```python
from build123d import *

# Parameters (mm, degrees)
EXTRUDE1_DEPTH     = 23.8125
SKETCH8_R          = 3.5687
CUT_EXTRUDE7_DEPTH = 73.566916507
SKETCH9_R          = 3.5687
CUT_EXTRUDE8_DEPTH = 73.566916507


with BuildPart() as part:
    # Sketch1 → Extrude1 (new, symmetric)
    with BuildSketch(Plane.XY):
        with BuildLine():
            Line((0, 0), (0, 50.8))
            ThreePointArc((0, 50.8), (-3.376576302, 49.401376302), (-4.7752, 46.0248))
            Line((-4.7752, 46.0248), (-4.7752, 8.3566))
            ThreePointArc((-4.7752, 8.3566), (-5.824167774, 5.824167774), (-8.3566, 4.7752))
            Line((-8.3566, 4.7752), (-46.0248, 4.7752))
            ThreePointArc((-46.0248, 4.7752), (-49.401376302, 3.376576302), (-50.8, 0))
            Line((-50.8, 0), (0, 0))
        make_face()
    extrude(amount=EXTRUDE1_DEPTH, both=True)

    # Sketch8 → Cut-Extrude7 (cut, through all)
    with BuildSketch(Plane(origin=(0, 4.7752, 0), x_dir=(1, 0, 0), z_dir=(0, 1, 0))):
        with Locations(Location((-38.1, -12.7, 0), (0, 0, 180))):
            Circle(SKETCH8_R)
        with Locations(Location((-12.7, -12.7, 0), (0, 0, 180))):
            Circle(SKETCH8_R)
        with Locations((-12.7, 12.7)):
            Circle(SKETCH8_R)
        with Locations((-38.1, 12.7)):
            Circle(SKETCH8_R)
    extrude(amount=-CUT_EXTRUDE7_DEPTH, mode=Mode.SUBTRACT)

    # Sketch9 → Cut-Extrude8 (cut, through all)
    with BuildSketch(Plane.ZY.offset(4.7752)):
        with Locations(Location((12.7, 12.7, 0), (0, 0, 270))):
            Circle(SKETCH9_R)
        with Locations(Location((12.7, 38.1, 0), (0, 0, 270))):
            Circle(SKETCH9_R)
        with Locations(Location((-12.7, 12.7, 0), (0, 0, 90))):
            Circle(SKETCH9_R)
        with Locations(Location((-12.7, 38.1, 0), (0, 0, 90))):
            Circle(SKETCH9_R)
    extrude(amount=-CUT_EXTRUDE8_DEPTH, mode=Mode.SUBTRACT)


solid = part.part
```
The model under review builds one solid part; all positions refer to its coordinate system, in mm. A direction names the side the tool comes from. Coordinates: 2 decimals unless noted, no trailing zeros. Write each loop counter-clockwise with the first axis right and the second up, starting at its lowest first coordinate (ties: lowest second). Pieces come first, ordered by that corner, then holes. Notation, with made-up numbers: (75.5, -38) -> (104.5, -38) arc R18 ccw to (104.5, -18) -> close; hole circle Ø2 at (59.5, 59). An arc over 180 degrees is marked (long way). One line per item, written item: value. Start each with the question number.
Q1. Clearance check with flat-ended pins moving along their axes: P1, Ø19, axis at x = -25, z = -5, coming from the +Y side; P2, Ø11.5, axis at y = 38.1, z = -12.7, coming from the -X side; P3, Ø2, axis at x = -7.5, z = 3.5, coming from the +Y side. State where each tip first meets the part, or that it passes through.
Q2. Add section B-B, the plane x = -38.1. Give the boundary of the cut face in (y, z).
Q3. The part is to be moulded in two halves that separate along X. For faces 3 (the face through (-34.803, 2.421, -11.333)), 4 (the face through (-14, 3, 23.812)), 5 (the face through (-3.34, 49.44, 0.33)), 6 (the face through (-37.326, 2.421, 9.216)), say which applies: +X half, -X half, draft (parallel to the pull), parting line (faces both ways), or undercut.
Q4. To check wall thickness, follow probe 1 along Z at (x, y) = (-2.75, 12.7); probe 2 along X at (y, z) = (3, 12); probe 3 along X at (y, z) = (2, 12). State the ranges of each line that lie inside material, in increasing order.
Q5. For faces 1 (the face through (-27, 4.775, 0)), 2 (the face through (-2.421, 15.532, 10.529)), list the 3-axis set-ups (+Z, -Z, +X, -X, +Y, -Y) from which the entire face can be reached by the end or side of a thin tool; tool diameter is ignored.
Q6. Add section D-D, the plane z = -3. Give the boundary of the cut face in (x, y).
Q7. Add section A-A, the plane y = 12.7. Give the boundary of the cut face in (x, z).
Q8. Add section C-C, the plane z = -12.7. Give the boundary of the cut face in (x, y).
Response:
1. P1: y = 4.78
1. P2: x = -4.78
1. P3: y = 5.29
2. outline: (0, -23.81) -> (4.78, -23.81) -> (4.78, -16.27) -> (0, -16.27) -> close; (0, -9.13) -> (4.78, -9.13) -> (4.78, 9.13) -> (0, 9.13) -> close; (0, 16.27) -> (4.78, 16.27) -> (4.78, 23.81) -> (0, 23.81) -> close
3. face 3: undercut
3. face 4: draft
3. face 5: -X half
3. face 6: undercut
4. probe 1: -23.81 to -16.27, -9.13 to 9.13, 16.27 to 23.81
4. probe 2: -49.74 to -41.6, -34.6 to -16.2, -9.2 to 0
4. probe 3: -50.36 to -41.6, -34.6 to -16.2, -9.2 to 0
5. face 1: +Z, -Z, -X, +Y
5. face 2: +X, -X
6. outline: (-50.8, 0) -> (0, 0) -> (0, 50.8) arc R4.78 ccw to (-4.78, 46.02) -> (-4.78, 8.36) arc R3.58 cw to (-8.36, 4.78) -> (-46.02, 4.78) arc R4.78 ccw to start
7. outline: (-4.78, -23.81) -> (0, -23.81) -> (0, -16.27) -> (-4.78, -16.27) -> close; (-4.78, -9.13) -> (0, -9.13) -> (0, 9.13) -> (-4.78, 9.13) -> close; (-4.78, 16.27) -> (0, 16.27) -> (0, 23.81) -> (-4.78, 23.81) -> close
8. outline: (-50.8, 0) -> (-41.67, 0) -> (-41.67, 4.78) -> (-46.02, 4.78) arc R4.78 ccw to start; (-34.53, 0) -> (-16.27, 0) -> (-16.27, 4.78) -> (-34.53, 4.78) -> close; (-9.13, 0) -> (0, 0) -> (0, 9.13) -> (-4.78, 9.13) -> (-4.78, 8.36) arc R3.58 cw to (-8.36, 4.78) -> (-9.13, 4.78) -> close; (-4.78, 16.27) -> (0, 16.27) -> (0, 34.53) -> (-4.78, 34.53) -> close; (-4.78, 41.67) -> (0, 41.67) -> (0, 50.8) arc R4.78 ccw to (-4.78, 46.02) -> close
